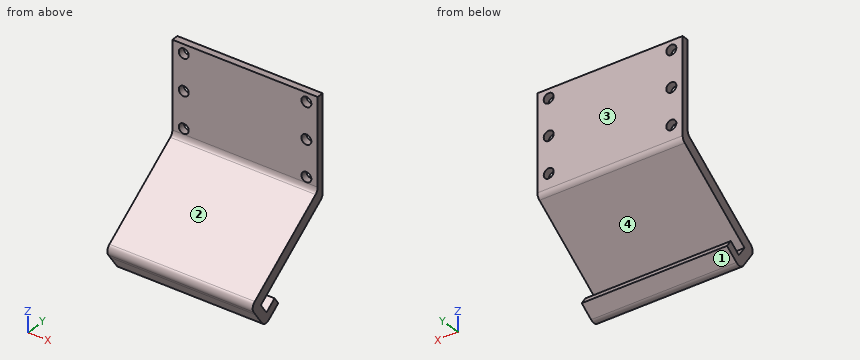
```python
from build123d import *

# Parameters (mm, degrees)
F0_W     = 64
F0_H     = 40
F0_R     = 2.2
F1_DEPTH = 3
F3_DEPTH = 32
F4_R     = 3


with BuildPart() as f1:
    # F0 (on Front) → F1 (new body)
    with BuildSketch(Plane.XZ):
        Rectangle(F0_W, F0_H)
        with Locations((-27, -16)):
            Circle(F0_R, mode=Mode.SUBTRACT)
        with Locations((27, -16)):
            Circle(F0_R, mode=Mode.SUBTRACT)
        with Locations((-27, 0)):
            Circle(F0_R, mode=Mode.SUBTRACT)
        with Locations((-27, 16)):
            Circle(F0_R, mode=Mode.SUBTRACT)
        with Locations((27, 0)):
            Circle(F0_R, mode=Mode.SUBTRACT)
        with Locations((27, 16)):
            Circle(F0_R, mode=Mode.SUBTRACT)
    extrude(amount=F1_DEPTH)

    # F2 (on Right) → F3 (join, symmetric)
    with BuildSketch(Plane.YZ):
        Polygon((0, -20), (-3, -20), (-43.8254843962, -48.5863119253), (-40.9576022144, -52.6820721467), (-37.6809940373, -50.3877664013), (0, -24.0032503292), align=None)
        Polygon((-37.6809940373, -50.3877664013), (-40.9576022144, -52.6820721467), (-35.2218378509, -60.8735925896), (-27.030317408, -55.1378282261), (-29.3246231535, -51.861220049), (-34.2395354192, -55.3026786671), align=None)
    extrude(amount=F3_DEPTH, both=True)

    # F4
    f4_edges = [f1.edges().sort_by_distance(p)[0] for p in [
        (0, -3, -20),
        (0, 0, -24.00325),
        (0, -43.825484, -48.586312),
        (0, -35.221838, -60.873593),
    ]]
    fillet(f4_edges, radius=F4_R)


solid = f1.part
```
Verification items for the finished model (mm, model axes). Face numbers are marked on the shaded views. Coordinates: 2 decimals unless noted, no trailing zeros. Loops run counter-clockwise (first coordinate to the right, second up) from the corner with the lowest first, then second, coordinate; pieces in that order, holes last. Notation, with made-up numbers: (-0.5, -28) -> (43.5, -28) arc R26 cw to (43.5, 2) -> close; hole circle Ø7 at (-24.5, 63.25). An arc over 180 degrees is marked (long way). Answer in a Markdown table with one row per item. Add a question column.
1. Material ranges on probe 1 along Z at (x, y) = (27, -1); probe 2 along Z at (x, y) = (-27, -1.95); probe 3 along Z at (x, y) = (26.5, -36), recorded low to high. Write a range as [from, to].
2. Section check A-A, the plane z = 16. Enter the section's corners in (x, y), then the cut area to 3 significant figures.
3. Draft check along Z on the marked faces 1, 2, 3 and 4. Enter one of: +Z half, -Z half, draft (parallel to the pull), parting line (faces both ways), or undercut.
4. Section check B-B, the plane x = -27. Enter the section's corners in (y, z), then the cut area to 3 significant figures.
5. Section check C-C, the plane x = -6.5. Enter the section's corners in (y, z), then the cut area to 3 significant figures.
6. Depth check by flat-ended pin: P1, Ø10, axis at x = -22, y = -24, coming from the -Z side; P2, Ø11.5, axis at x = -4.5, z = -2.5, coming from the -Y side; P3, Ø4, axis at x = 27, z = 0, coming from the -Y side; P4, Ø7, axis at x = -27, z = 0, coming from the +Y side. Enter the tip coordinate at first touch or a pass-through.
7. Section check D-D, the plane x = 26. Enter the section's corners in (y, z).
Derived:
| question | item | result |
|---|---|---|
| 1 | probe 1 | z = [-24.68, -18.2], [-13.8, -2.2], [2.2, 13.8], [18.2, 20] |
| 1 | probe 2 | z = [-25.37, -18.2], [-13.8, -2.2], [2.2, 13.8], [18.2, 20] |
| 1 | probe 3 | z = [-59.28, -52.79], [-49.21, -43.11] |
| 2 | outline | (-32, -3) -> (-29.2, -3) -> (-29.2, 0) -> (-32, 0) -> close; (-24.8, -3) -> (24.8, -3) -> (24.8, 0) -> (-24.8, 0) -> close; (29.2, -3) -> (32, -3) -> (32, 0) -> (29.2, 0) -> close |
| 2 | area | 166 mm² |
| 3 | face 1 | -Z half |
| 3 | face 2 | +Z half |
| 3 | face 3 | draft |
| 3 | face 4 | undercut |
| 4 | outline | (-42.1, -51.04) -> (-36.94, -58.42) arc R3 ccw to (-32.76, -59.15) -> (-27.03, -55.14) -> (-29.32, -51.86) -> (-34.24, -55.3) -> (-37.68, -50.39) -> (-1.28, -24.9) arc R3 ccw to (0, -22.44) -> (0, -18.2) -> (-3, -18.2) -> (-3, -18.44) arc R3 cw to (-4.28, -20.9) -> (-41.37, -46.87) arc R3 ccw to start; (-3, -13.8) -> (0, -13.8) -> (0, -2.2) -> (-3, -2.2) -> close; (-3, 2.2) -> (0, 2.2) -> (0, 13.8) -> (-3, 13.8) -> close; (-3, 18.2) -> (0, 18.2) -> (0, 20) -> (-3, 20) -> close |
| 4 | area | 396 mm² |
| 5 | outline | (-42.1, -51.04) -> (-36.94, -58.42) arc R3 ccw to (-32.76, -59.15) -> (-27.03, -55.14) -> (-29.32, -51.86) -> (-34.24, -55.3) -> (-37.68, -50.39) -> (-1.28, -24.9) arc R3 ccw to (0, -22.44) -> (0, 20) -> (-3, 20) -> (-3, -18.44) arc R3 cw to (-4.28, -20.9) -> (-41.37, -46.87) arc R3 ccw to start |
| 5 | area | 436 mm² |
| 6 | P1 | stops at z = -56.52 |
| 6 | P2 | stops at y = -3 |
| 6 | P3 | passes through |
| 6 | P4 | stops at y = 0 |
| 7 | outline | (-42.1, -51.04) -> (-36.94, -58.42) arc R3 ccw to (-32.76, -59.15) -> (-27.03, -55.14) -> (-29.32, -51.86) -> (-34.24, -55.3) -> (-37.68, -50.39) -> (-1.28, -24.9) arc R3 ccw to (0, -22.44) -> (0, -17.96) -> (-3, -17.96) -> (-3, -18.44) arc R3 cw to (-4.28, -20.9) -> (-41.37, -46.87) arc R3 ccw to start; (-3, -14.04) -> (0, -14.04) -> (0, -1.96) -> (-3, -1.96) -> close; (-3, 1.96) -> (0, 1.96) -> (0, 14.04) -> (-3, 14.04) -> close; (-3, 17.96) -> (0, 17.96) -> (0, 20) -> (-3, 20) -> close |
